Build history of the part. All positions in model axes, mm. A direction names the side the tool comes from. Give positions to 0.01 mm unless a question says otherwise; leave off trailing zeros. Order: outer loops, then holes, each group sorted by start corner. A loop starts at its lowest first (then second) coordinate and runs counter-clockwise, first axis right, second up. Notation, with made-up numbers: M -13.5,71.5 L 20.5,71.5 A20 cw 20.5,102.5 Z; hole C 51,-3 d5. An arc over 180 degrees is marked long. One line per item, written item: value. Start each with the question number.
from build123d import *

# Parameters (mm, degrees)
SKETCH1_R           = 1.65
BOSS_EXTRUDE1_DEPTH = 2


with BuildPart() as part:
    # Sketch1 → Boss-Extrude1 (new body)
    with BuildSketch(Plane.XY):
        with BuildLine():
            Line((7.72, -4), (0, -4))
            ThreePointArc((0, -4), (-2.529822128, -3.098386677), (-3.919183588, -0.8))
            Line((-3.919183588, -0.8), (-8.919183588, -0.8))
            Line((-8.919183588, -0.8), (-8.919183588, 1.2))
            Line((-8.919183588, 1.2), (-3.919183588, 1.2))
            Line((-3.919183588, 1.2), (-3.919183588, 3.2))
            Line((-3.919183588, 3.2), (-2.4, 3.2))
            ThreePointArc((-2.4, 3.2), (0.404610957, 3.979483631), (2.994944065, 2.651473185))
            Line((2.994944065, 2.651473185), (2.994944065, -1.348526815))
            Line((2.994944065, -1.348526815), (7.72, -1.348526815))
            Line((7.72, -1.348526815), (7.72, -4))
        make_face()
        Circle(SKETCH1_R, mode=Mode.SUBTRACT)
    extrude(amount=BOSS_EXTRUDE1_DEPTH)


solid = part.part
1) Drill centre lines: line 1 (Y direction, x = 0, z = 0.55); line 2 (Y direction, x = 4, z = 1.9); line 3 (Y direction, x = -4.75, z = 1.7). Where is each one in solid material? Low to high.
2) Slice it at D-D (x = 4.5). List the corners of the cut face in (y, z), plus the area to 3 significant figures.
3) Pull direction Y, two halves, no side cores. Call faces 4 (the flat face through (4, -4, 1)), 5 (the cylindrical face through (-1.216, 1.115, 0.986)), 6 (the flat face through (-3.919, 2, 1)), 7 (the flat face through (5, -1.349, 1)): pulls with the +Y half, pulls with the -Y half, needs draft (parallel to the pull), parting line crosses it, or undercut.
4) Slice it at A-A (z = 0.2). List the corners of the cut face in (x, y), plus the area to 3 significant figures.
5) Slice it at C-C (x = 1). List the corners of the cut face in (y, z).
6) Drop flat-ended pins along their axis: P1, Ø1, axis at x = 5.5, z = 1, coming from the +Y side; P2, Ø0.5, axis at x = -3, z = 1, coming from the +Y side; P3, Ø0.6, axis at x = -7, z = 1, coming from the -Y side. Give the stop position or say it passes through.
7) Slice it at B-B (y = 0). List the corners of the cut face in (x, z).
8) Tool access for faces 1 (the flat face through (2.995, 1, 1)), 2 (the flat face through (-6, -0.8, 1)), 3 (the flat face through (-6, 1.2, 1)): list every direction of +Z, -Z, +X, -X, +Y, -Y with a clear straight run to the whole face (end or side of a thin tool).
Results list:
1. line 1: y = -4 to -1.65, 1.65 to 4
1. line 2: y = -4 to -1.35
1. line 3: y = -0.8 to 1.2
2. outline: M -4,0 L -1.35,0 L -1.35,2 L -4,2 Z
2. area: 5.30 mm²
3. face 4: pulls with the -Y half
3. face 5: undercut
3. face 6: needs draft
3. face 7: pulls with the +Y half
4. outline: M -8.92,-0.8 L -3.92,-0.8 A4 ccw 0,-4 L 7.72,-4 L 7.72,-1.35 L 2.99,-1.35 L 2.99,2.65 A4 ccw -2.4,3.2 L -3.92,3.2 L -3.92,1.2 L -8.92,1.2 Z; hole C 0,0 d3.3
4. area: 63.1 mm²
5. outline: M -4,0 L -1.31,0 L -1.31,2 L -4,2 Z; M 1.31,0 L 3.87,0 L 3.87,2 L 1.31,2 Z
6. P1: stops at y = -1.35
6. P2: stops at y = 3.2
6. P3: stops at y = -0.8
7. outline: M -8.92,0 L -1.65,0 L -1.65,2 L -8.92,2 Z; M 1.65,0 L 2.99,0 L 2.99,2 L 1.65,2 Z
8. face 1: +Z, -Z, +X, +Y
8. face 2: +Z, -Z, -X, -Y
8. face 3: +Z, -Z, -X, +Y
